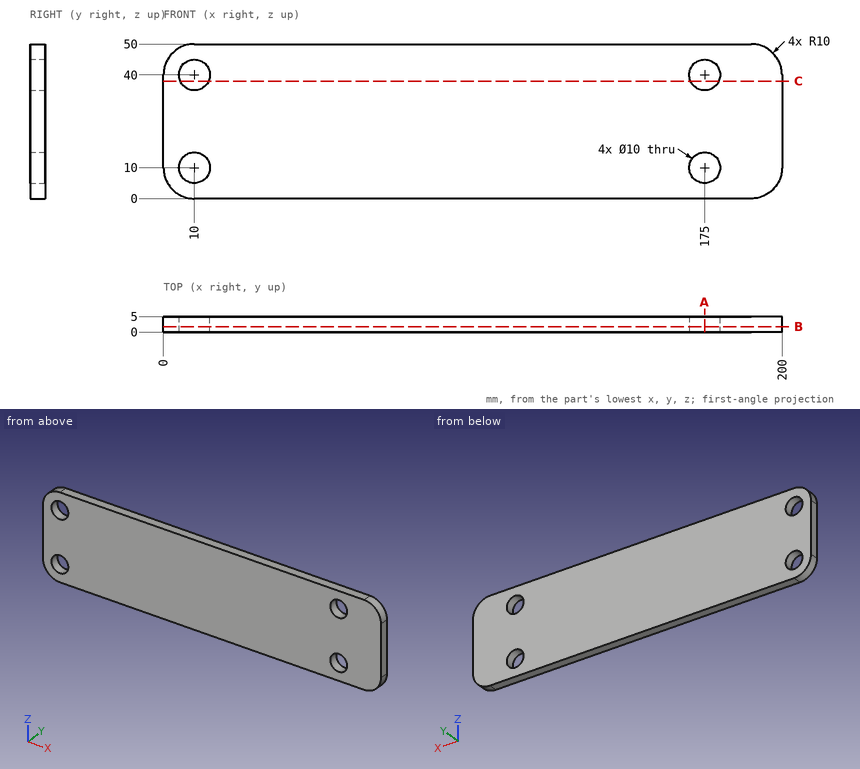
Geometry check sheet. Reference: drawing and pictorial views, mm from the part's lowest x, y, z. Give positions to 0.01 mm unless a question says otherwise; leave off trailing zeros. Loops run counter-clockwise (first coordinate to the right, second up) from the corner with the lowest first, then second, coordinate; pieces in that order, holes last. Notation, with made-up numbers: M 41.5,74.5 L 53.5,74.5 A23 ccw 53.5,82.5 Z; hole C 89.5,-3.75 d3. An arc over 180 degrees is marked long. Use a Markdown table: item, result. Add a question column.
Q1. Sectioned sample at B-B, the plane y = 1.8. Record the cut outline in (x, z).
Q2. Scan lines: line 1 along Z through (x, y) = (10, 2.1); line 2 along X through (y, z) = (3.3, 6). Record each from-to range of solid material in increasing order. Write a range as [from, to].
Q3. Go/stop test with a flat-tipped pin: pin 1 (8 mm diameter, centred on x = 175, z = 40, fed in from +Y). Record where the tip stops, or that it passes through.
Q4. Sectioned sample at A-A, the plane x = 175. Record the cut outline in (y, z).
Q5. Sectioned sample at C-C, the plane z = 38. Record the cut outline in (x, y).
Verdict:
| question | item | result |
|---|---|---|
| 1 | outline | M 0,10 A10 ccw 10,0 L 190,0 A10 ccw 200,10 L 200,40 A10 ccw 190,50 L 10,50 A10 ccw 0,40 Z; hole C 10,10 d10; hole C 10,40 d10; hole C 175,10 d10; hole C 175,40 d10 |
| 2 | line 1 | [0, 5], [15, 35], [45, 50] |
| 2 | line 2 | [0.83, 7], [13, 172], [178, 199.17] |
| 3 | pin 1 | through |
| 4 | outline | M 0,0 L 5,0 L 5,5 L 0,5 Z; M 0,15 L 5,15 L 5,35 L 0,35 Z; M 0,45 L 5,45 L 5,50 L 0,50 Z |
| 5 | outline | M 0,0 L 5.42,0 L 5.42,5 L 0,5 Z; M 14.58,0 L 170.42,0 L 170.42,5 L 14.58,5 Z; M 179.58,0 L 200,0 L 200,5 L 179.58,5 Z |
